Geometry check sheet. Reference: the model listing, model coordinates, mm. Give positions to 0.01 mm unless a question says otherwise; leave off trailing zeros. Write each loop counter-clockwise with the first axis right and the second up, starting at its lowest first coordinate (ties: lowest second). Pieces come first, ordered by that corner, then holes. Notation, with made-up numbers: (37, 59) -> (54, 59) arc R28 ccw to (54, 79) -> close; hole circle Ø3 at (82.25, 85.5). An arc over 180 degrees is marked (long way). Write item = value, one per line. Start each with the question number.
1. Thickness scan on line 1 along X through (y, z) = (138.5, -75.5); line 2 along Y through (x, z) = (-139, -73.75). Record the ranges inside material, lowest first.
2. Cross-section at B-B, the plane y = 66. Record the cut outline in (x, z).
3. Cross-section at A-A, the plane x = -179. Record the cut outline in (y, z).
4. Depth check by flat-ended pin: P1, Ø3, axis at x = -3, z = -74.5, coming from the +Y side; P2, Ø1.9, axis at y = -2, z = -75.5, coming from the -X side; P3, Ø1, axis at x = -103.5, z = -73, coming from the -Y side. Enter the tip coordinate at first touch or a pass-through.
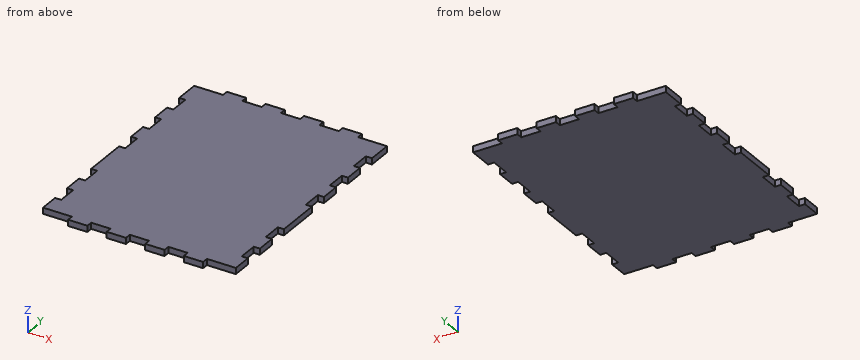
```python
from build123d import *

# Parameters (mm, degrees)
BOSS_EXTRUDE1_DEPTH = 6.35


with BuildPart() as part:
    # Sketch1 → Boss-Extrude1 (new body)
    with BuildSketch(Plane(origin=(0, 0, -77.734937154), x_dir=(-1, 0, 0), z_dir=(0, 0, -1))):
        Polygon((0, 80), (6.35, 80), (6.35, 60), (0, 60), (0, 40), (6.35, 40), (6.35, 20), (0, 20), (0, 0), (30, 0), (30, -6.35), (50, -6.35), (50, 0), (70, 0), (70, -6.35), (90, -6.35), (90, 0), (110, 0), (110, -6.35), (130, -6.35), (130, 0), (150, 0), (150, -6.35), (170, -6.35), (170, 0), (200, 0), (200, 20), (193.65, 20), (193.65, 40), (200, 40), (200, 60), (193.65, 60), (193.65, 80), (200, 80), (200, 126.5875), (193.65, 126.5875), (193.65, 146.5875), (200, 146.5875), (200, 166.5875), (193.65, 166.5875), (193.65, 186.5875), (200, 186.5875), (200, 206.5875), (193.65, 206.5875), (193.65, 226.5875), (200, 226.5875), (200, 251.5875), (170, 251.5875), (170, 257.9375), (150, 257.9375), (150, 251.5875), (130, 251.5875), (130, 257.9375), (110, 257.9375), (110, 251.5875), (90, 251.5875), (90, 257.9375), (70, 257.9375), (70, 251.5875), (50, 251.5875), (50, 257.9375), (30, 257.9375), (30, 251.5875), (0, 251.5875), (0, 226.5875), (6.35, 226.5875), (6.35, 206.5875), (0, 206.5875), (0, 186.5875), (6.35, 186.5875), (6.35, 166.5875), (0, 166.5875), (0, 146.5875), (6.35, 146.5875), (6.35, 126.5875), (0, 126.5875), align=None)
    extrude(amount=-BOSS_EXTRUDE1_DEPTH)


solid = part.part
```
Answers:
q1.line_1 = -193.65 to -6.35
q1.line_2 = 0 to 251.59
q2.outline = (-193.65, -77.73) -> (-6.35, -77.73) -> (-6.35, -71.38) -> (-193.65, -71.38) -> close
q3.outline = (0, -77.73) -> (251.59, -77.73) -> (251.59, -71.38) -> (0, -71.38) -> close
q4.P1 = 251.59
q4.P2 = -170
q4.P3 = 0
